Here's the drawing with two shaded views (mm, measured from the low corner). I have some questions. A direction names the side the tool comes from. Round coordinates to 2 decimals unless told otherwise and drop trailing zeros. Loops run counter-clockwise (first coordinate to the right, second up) from the corner with the lowest first, then second, coordinate; pieces in that order, holes last. Notation, with made-up numbers: (51.5, -2.5) -> (92.5, -2.5) arc R28 ccw to (92.5, 17.5) -> close; hole circle Ø5 at (9, -19.5). An arc over 180 degrees is marked (long way). Write item = value, one per line.
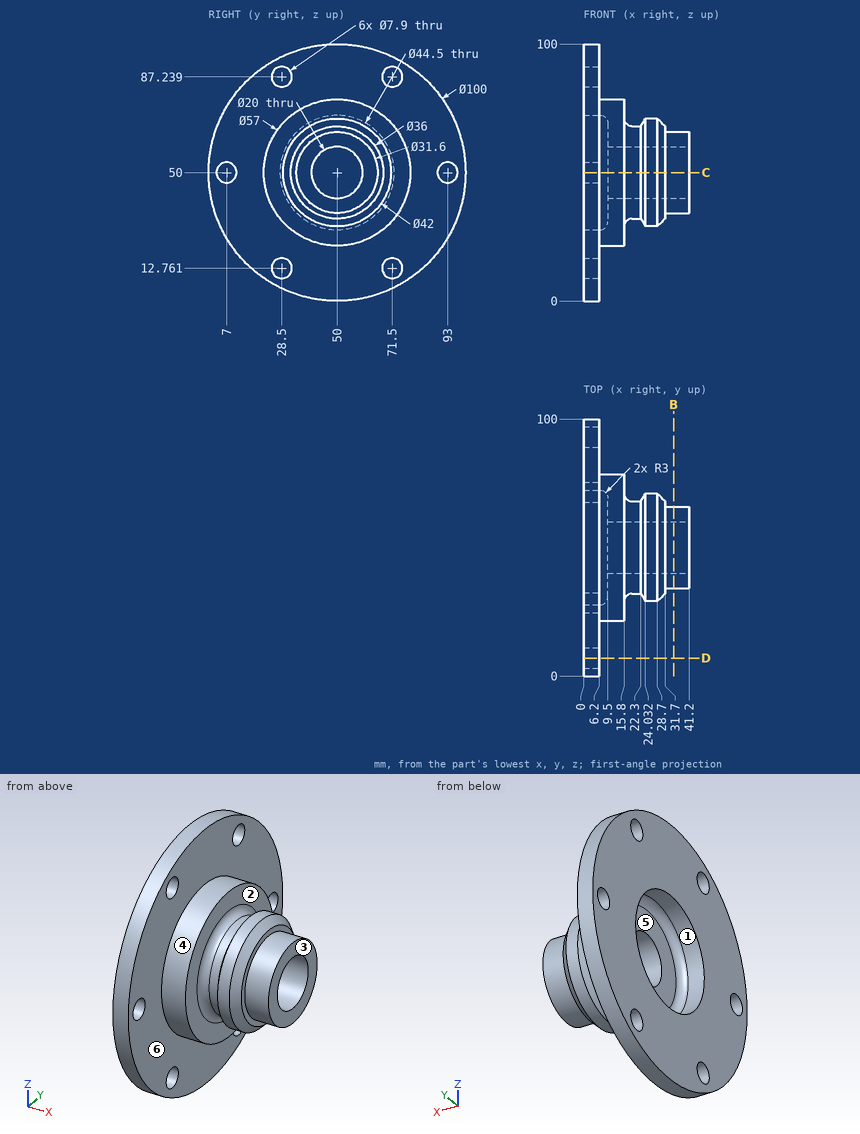
1. I need wall thicknesses on line 1 (Y direction, x = 5.25, z = 50); line 2 (Y direction, x = 20.5, z = 50); line 3 (X direction, y = 54.5, z = 12). Which ranges of each line are inside material? Lowest first, please. Write a range as [from, to].
Entries:
line_1 = [0, 3.05], [10.95, 27.75], [72.25, 89.05], [96.95, 100]
line_2 = [32, 40], [60, 68]
line_3 = [0, 6.2]
2. I'm going to push flat-ended pins straight in: pin 1 (1 mm diameter, centred on x = 36, z = 62.5, fed in from +Y); pin 2 (11.5 mm diameter, centred on y = 42.5, z = 45.5, fed in from -X); pin 3 (4.5 mm diameter, centred on y = 28.5, z = 87.24, fed in from -X); pin 4 (8 mm diameter, centred on x = 31, z = 42.5, fed in from +Y). Where does each tip first touch, or does it pass through?
Entries:
pin_1 = 60.28
pin_2 = 9.5
pin_3 = through
pin_4 = 70.57
3. Suppose I cut it at C-C, the plane z = 50. Count the separate pieces of the cut face and the enclosed holes in it, and give its area (3 significant figures).
Entries:
separate_pieces = 4
enclosed_holes = 0
area = 935 mm²
4. Suppose I cut it at D-D, the plane y = 7. List the corners of the cut face in (x, z) for me.
Entries:
outline = (0, 24.49) -> (6.2, 24.49) -> (6.2, 46.05) -> (0, 46.05) -> close; (0, 53.95) -> (6.2, 53.95) -> (6.2, 75.51) -> (0, 75.51) -> close
5. We'd pull the mould along Y, two halves only. Please class the marked faces 4, 5 and 6: released by +Y, released by -Y, zero draft, split by the parting line, or undercut.
Entries:
face_4 = split by the parting line
face_5 = undercut
face_6 = zero draft
6. Suppose I cut it at B-B, the plane x = 35. List the corners of the cut face in (y, z) for me, and give its area (3 significant figures).
Entries:
outline = circle Ø31.6 at (50, 50); hole circle Ø20 at (50, 50)
area = 470 mm²
7. For the marked faces 1, 2 and 3, which set-ups out of +Z, -Z, +X, -X, +Y, -Y let a thin tool reach every point of the face, with its end or its side?
Entries:
face_1 = -X
face_2 = +X
face_3 = +Z, -Z, +X, +Y, -Y
